Work out the finished part from the listing and answer in its coordinate system (mm). Face numbers are marked on the shaded views. A direction names the side the tool comes from. Give positions to 0.01 mm unless a question says otherwise; leave off trailing zeros. Loops run counter-clockwise (first coordinate to the right, second up) from the corner with the lowest first, then second, coordinate; pieces in that order, holes last.
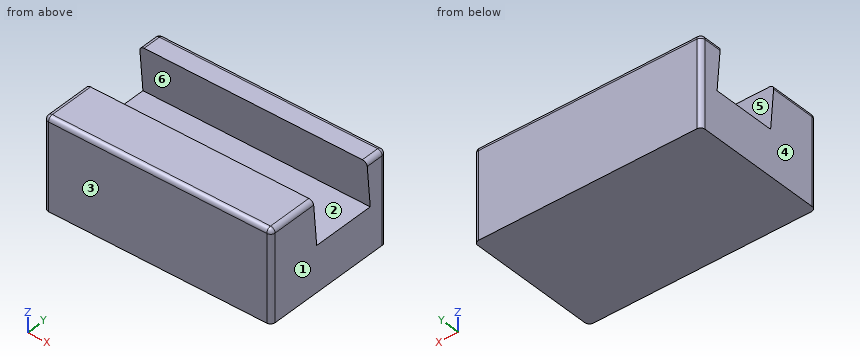
```python
from build123d import *

# Parameters (mm, degrees)
F0_W     = 30
F0_H     = 20
F1_DEPTH = 25
F3_DEPTH = 50
F4_R     = 1


with BuildPart() as f1:
    # F0 (on Right) → F1 (new body, symmetric)
    with BuildSketch(Plane.YZ):
        with Locations((0, 10)):
            Rectangle(F0_W, F0_H)
    extrude(amount=F1_DEPTH, both=True)

    # F2 (on face) → F3 (cut)
    with BuildSketch(Plane.YZ.offset(25)):
        Polygon((10.874887, 10), (10, 20), (-4, 20), (-3.125113, 10), align=None)
    extrude(amount=-F3_DEPTH, mode=Mode.SUBTRACT)

    # F4
    f4_edges = [f1.edges().sort_by_distance(p)[0] for p in [
        (0, -15, 20),
        (25, -9.5, 20),
        (25, 12.5, 20),
        (0, 15, 20),
        (25, 15, 10),
        (25, -15, 10),
        (-25, -15, 10),
        (-25, -9.5, 20),
        (-25, 12.5, 20),
        (-25, 15, 10),
    ]]
    fillet(f4_edges, radius=F4_R)


solid = f1.part
```
Q1. Given pin 1 (3 mm diameter, centred on x = 9, y = 1, fed in from -Z); pin 2 (7 mm diameter, centred on x = -3, y = 0.5, fed in from +Z), each flat-ended and moving along its own axis, determine where each tip first touches the part or whether it passes through.
Q2. Consider line 1 along Z through (x, y) = (-16.5, 9.75); line 2 along Y through (x, z) = (-4, 12.25); line 3 along Y through (x, z) = (-17.5, 14.5). Determine where each line is inside the solid, lowest interval first.
Q3. Section C-C on y = 0.75 is taken. Give the vertices of the cut face in (x, z).
Q4. Section B-B on z = 17 is taken. Give the vertices of the cut face in (x, y).
Q5. Determine the mould class of the marked faces 1, 2 and 3 for opening direction Y: +Y half, -Y half, draft (parallel to the pull), parting line (faces both ways), or undercut.
Q6. Section A-A on x = 8.5 is taken. Give the vertices of the cut face in (y, z).
Q7. Which of the six approach directions +Z, -Z, +X, -X, +Y, -Y give full straight-line access (tool end or side, diameter ignored) to the marked faces 4, 5 and 6?
Check result:
1. pin 1: stops at z = 0
1. pin 2: stops at z = 10
2. line 1: z = 0 to 10
2. line 2: y = -15 to -3.32, 10.68 to 15
2. line 3: y = -15 to -3.52, 10.48 to 15
3. outline: (-25, 0) - (25, 0) - (25, 10) - (-25, 10) - close
4. outline: (-25, -14) arc R1 ccw to (-24, -15) - (24, -15) arc R1 ccw to (25, -14) - (25, -3.74) - (-25, -3.74) - close; (-25, 10.26) - (25, 10.26) - (25, 14) arc R1 ccw to (24, 15) - (-24, 15) arc R1 ccw to (-25, 14) - close
5. face 1: draft
5. face 2: undercut
5. face 3: -Y half
6. outline: (-15, 0) - (15, 0) - (15, 19) arc R1 ccw to (14, 20) - (10, 20) - (10.87, 10) - (-3.13, 10) - (-4, 20) - (-14, 20) arc R1 ccw to (-15, 19) - close
7. face 4: +Z, -Z, -X, +Y, -Y
7. face 5: +Z, +X, -X
7. face 6: +X, -X
